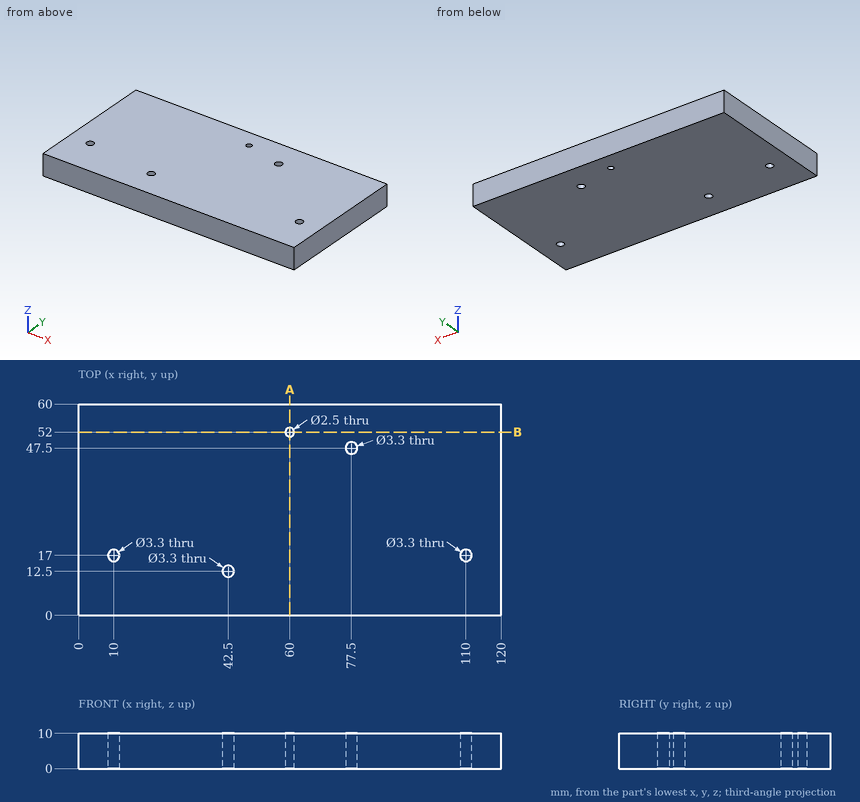
Design review of the part shown in the three views and the two pictorial views. Dimensions are in mm from the part's minimum x, y and z. Round coordinates to 2 decimals unless told otherwise and drop trailing zeros. Loops run counter-clockwise (first coordinate to the right, second up) from the corner with the lowest first, then second, coordinate; pieces in that order, holes last. Notation, with made-up numbers: (15.5, -28.5) -> (28.5, -28.5) arc R25 ccw to (28.5, 1.5) -> close; hole circle Ø8 at (71.5, 3.5). An arc over 180 degrees is marked (long way). Answer as CSV lines item,"result".
1) Add section B-B on y = 52. Write out the cut boundary in (x, z), plus the area to 4 significant figures.
Geometry results:
outline,"(0, 0) -> (58.75, 0) -> (58.75, 10) -> (0, 10) -> close; (61.25, 0) -> (120, 0) -> (120, 10) -> (61.25, 10) -> close"
area,"1,175 mm²"
2) For P1, Ø3, axis at x = 110, y = 17, coming from the -Z side, flat-tipped, find the tip position at first contact; note if it passes through.
Geometry results:
P1,"passes through"
3) Add section A-A on x = 60. Write out the cut boundary in (y, z), plus the area to 3 significant figures.
Geometry results:
outline,"(0, 0) -> (50.75, 0) -> (50.75, 10) -> (0, 10) -> close; (53.25, 0) -> (60, 0) -> (60, 10) -> (53.25, 10) -> close"
area,"575 mm²"
4) To check wall thickness, follow line 1 along Y through (x, z) = (110, 2.75); line 2 along Y through (x, z) = (42.5, 4.5); line 3 along X through (y, z) = (52, 2). State the ranges of each line that lie inside material, in increasing order. Write a range as from..to.
Geometry results:
line 1,"y = 0..15.35, 18.65..60"
line 2,"y = 0..10.85, 14.15..60"
line 3,"x = 0..58.75, 61.25..120"
